Design review of the part built by this model. Coordinates are the model's own, in mm. Coordinates: 2 decimals unless noted, no trailing zeros. Loops run counter-clockwise (first coordinate to the right, second up) from the corner with the lowest first, then second, coordinate; pieces in that order, holes last.
Q1. Add section B-B on y = 13.97. Give the boundary of the cut face in (x, z) (3 decimals).
Q2. Wall thickness on probe 1 along X at (y, z) = (0, 0.6) (3 decimals); probe 2 along Y at (x, z) = (0, 1.3) (3 decimals); probe 3 along Y at (x, z) = (13.97, 0.9) (3 decimals): over which ranges is each line inside the solid? List them lowest first.
Q3. Add section A-A on x = 0. Give the boundary of the cut face in (y, z) (3 decimals), and give its area (3 significant figures).
Q4. For P1, Ø1, axis at y = 4, z = 2.5, coming from the +X side; P2, Ø2.5, axis at x = -13.97, y = 0, coming from the +Z side; P3, Ø1.1, axis at x = -12.065, y = -20.955, coming from the +Z side; P4, Ø8, axis at x = -1.5, y = 7.5, coming from the -Z side, all flat-tipped, find the tip position at first contact; note any pin that passes through.
Q5. Add section D-D on y = 8.5. Give the boundary of the cut face in (x, z) (3 decimals), and give its area (3 significant figures).
Q6. Add section C-C on x = -9. Give the boundary of the cut face in (y, z) (3 decimals).
```python
from build123d import *

# Parameters (mm, degrees)
BOSS_EXTRUDE1_DEPTH                               = 3.175
CSK_FOR_0_FLAT_HEAD_SOCKET_CAP_SCREW1_D           = 1.778
CSK_FOR_0_FLAT_HEAD_SOCKET_CAP_SCREW1_CSINK_D     = 3.5052
CSK_FOR_0_FLAT_HEAD_SOCKET_CAP_SCREW1_CSINK_ANGLE = 82


with BuildPart() as part:
    # Sketch1 → Boss-Extrude1 (new body)
    with BuildSketch(Plane.XY):
        with BuildLine():
            Line((-15.875, 0), (-15.875, -28.575))
            Line((-15.875, -28.575), (15.875, -28.575))
            Line((15.875, -28.575), (15.875, 0))
            ThreePointArc((15.875, 0), (0, 15.875), (-15.875, 0))
        make_face()
    extrude(amount=BOSS_EXTRUDE1_DEPTH)

    # CSK for #0 Flat Head Socket Cap Screw1 (through all)
    with Locations(Plane.XY.offset(3.175)):
        with Locations((0, 13.97), (-13.97, 0), (13.97, 0), (-12.065, -20.955), (12.065, -20.955)):
            CounterSinkHole(CSK_FOR_0_FLAT_HEAD_SOCKET_CAP_SCREW1_D / 2, CSK_FOR_0_FLAT_HEAD_SOCKET_CAP_SCREW1_CSINK_D / 2, counter_sink_angle=CSK_FOR_0_FLAT_HEAD_SOCKET_CAP_SCREW1_CSINK_ANGLE)


solid = part.part
```
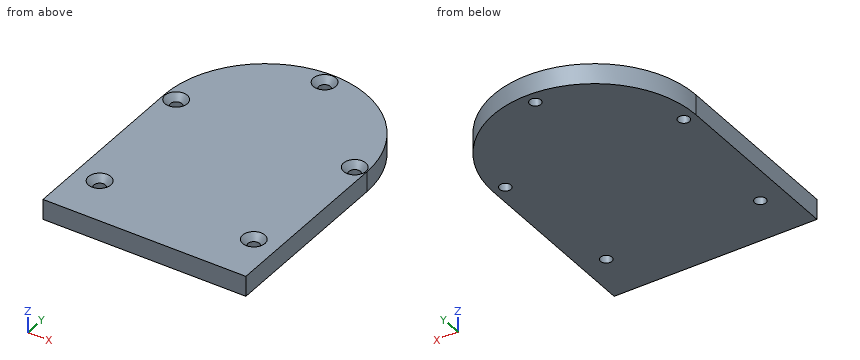
Entries:
1. outline: (-7.54, 0) - (-0.889, 0) - (-0.889, 2.182) - (-1.753, 3.175) - (-7.54, 3.175) - close; (0.889, 0) - (7.54, 0) - (7.54, 3.175) - (1.753, 3.175) - (0.889, 2.182) - close
2. probe 1: x = -15.875 to -14.859, -13.081 to 13.081, 14.859 to 15.875
2. probe 2: y = -28.575 to 13.081, 14.859 to 15.875
2. probe 3: y = -28.575 to -0.889, 0.889 to 7.54
3. outline: (-28.575, 0) - (13.081, 0) - (13.081, 2.182) - (12.217, 3.175) - (-28.575, 3.175) - close; (14.859, 0) - (15.875, 0) - (15.875, 3.175) - (15.723, 3.175) - (14.859, 2.182) - close
3. area: 135 mm2
4. P1: stops at x = 15.48
4. P2: stops at z = 2.6
4. P3: passes through
4. P4: stops at z = 0
5. outline: (-13.408, 0) - (13.408, 0) - (13.408, 3.175) - (-13.408, 3.175) - close
5. area: 85.1 mm2
6. outline: (-28.575, 0) - (13.077, 0) - (13.077, 3.175) - (-28.575, 3.175) - close
